from build123d import *

# Parameters (mm, degrees)
SKETCH1_R           = 4.7625
BOSS_EXTRUDE1_DEPTH = 7.1628
BOSS_EXTRUDE2_DEPTH = 44.45
BOSS_EXTRUDE3_START = 9.6774
SKETCH3_R           = 4.7625
BOSS_EXTRUDE3_DEPTH = 9.6774
CHAMFER1_SIZE       = 0.79375


with BuildPart() as part:
    # Sketch1 → Boss-Extrude1 (new body)
    with BuildSketch(Plane.XY):
        with Locations((8.861538462, 6.041958042)):
            Circle(SKETCH1_R)
    extrude(amount=-BOSS_EXTRUDE1_DEPTH)

    # Sketch2 → Boss-Extrude2 (add)
    with BuildSketch(Plane.XY):
        Polygon((13.624038462, 8.791588699), (8.861538462, 11.541219356), (4.099038462, 8.791588699), (4.099038462, 3.292327385), (8.861538462, 0.542696728), (13.624038462, 3.292327385), align=None)
    extrude(amount=BOSS_EXTRUDE2_DEPTH)

    # Sketch3 → Boss-Extrude3 (add)
    with BuildSketch(Plane.XY.offset(44.45).offset(BOSS_EXTRUDE3_START)):
        with Locations((8.861538462, 6.041958042)):
            Circle(SKETCH3_R)
    extrude(amount=-BOSS_EXTRUDE3_DEPTH)

    # Chamfer1
    chamfer1_edges = [part.edges().sort_by_distance(p)[0] for p in [
        (4.099038462, 6.041958042, 54.1274),
        (4.099038462, 6.041958042, -7.1628),
    ]]
    chamfer(chamfer1_edges, length=CHAMFER1_SIZE)


solid = part.part
CAD build for the part. Positions are in the model's coordinates, mm. A direction names the side the tool comes from. Round coordinates to 2 decimals unless told otherwise and drop trailing zeros. Loops run counter-clockwise (first coordinate to the right, second up) from the corner with the lowest first, then second, coordinate; pieces in that order, holes last.
(1) Wall check: line 1 along Y through (x, z) = (11.5, 5.5); line 2 along Y through (x, z) = (8, 18.5); line 3 along Z through (x, y) = (6.5, 9.75). Give the ranges that are in metal, low to high.
(2) Which spindle directions (+Z, -Z, +X, -X, +Y, -Y) get a long thin tool onto all of the face, cutting with end or side? Do faces 1 (the flat face through (9, 1, 0)), 2 (the flat face through (4.6, 3.5, 0)), 3 (the flat face through (4.6, 8.6, 44.45)). Say none if no direction does.
(3) Cut at A-A (z = 50.5). Give the cut face in (x, y) (1 decimal).
(4) Drop flat-ended pins along their axis: pin 1 (0.7 mm diameter, centred on x = 5.5, y = 9, fed in from -Z); pin 2 (0.7 mm diameter, centred on x = 13, y = 3.5, fed in from +Z); pin 3 (2 mm diameter, centred on y = 2, z = 16, fed in from -X). Give the stop position or say it passes through.
(5) Cut at B-B (z = 20). Give the cut face in (x, y), plus the area to 3 significant figures.
Findings below:
1. line 1: y = 2.07 to 10.02
1. line 2: y = 1.04 to 11.04
1. line 3: z = -6.74 to 53.7
2. face 1: -Z, -Y
2. face 2: -Z, -X, -Y
2. face 3: +Z, -X, +Y
3. outline: circle Ø9.5 at (8.9, 6)
4. pin 1: stops at z = -7
4. pin 2: stops at z = 53.59
4. pin 3: stops at x = 4.61
5. outline: (4.1, 3.29) - (8.86, 0.54) - (13.62, 3.29) - (13.62, 8.79) - (8.86, 11.54) - (4.1, 8.79) - close
5. area: 78.6 mm2
